The model under review builds one solid part; all positions refer to its coordinate system, in mm. Face numbers are marked on the shaded views. A direction names the side the tool comes from. Coordinates: 2 decimals unless noted, no trailing zeros. Loops run counter-clockwise (first coordinate to the right, second up) from the corner with the lowest first, then second, coordinate; pieces in that order, holes last. Notation, with made-up numbers: M 64,-5 L 73,-5 A35 cw 73,34 Z; hole C 2,8.5 d6. An arc over 180 degrees is marked long. Return JSON: item names as keys, results as strings.
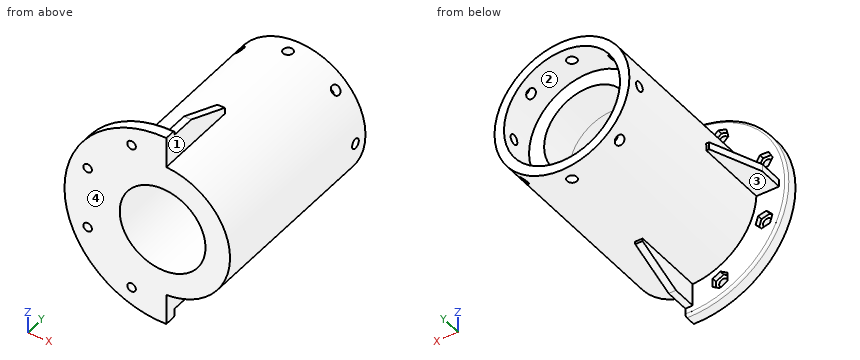
```python
from build123d import *

# Parameters (mm, degrees)
SKETCH1_R                = 27.5
SKETCH1_R_2              = 23.65
BOSS_EXTRUDE1_DEPTH      = 30
SKETCH2_R                = 2
CUT_EXTRUDE1_DEPTH       = 28.5
CIRPATTERN1_COUNT        = 4
CIRPATTERN1_ANGLE        = 135
SKETCH3_R                = 27.5
SKETCH3_R_2              = 23.65
BOSS_EXTRUDE2_DEPTH      = 51
BOSS_EXTRUDE3_DEPTH      = 5
SKETCH6_W                = 3
SKETCH6_H                = 12
SKETCH6_W_2              = 12
SKETCH6_H_2              = 3
BOSS_EXTRUDE4_DEPTH      = 30
CHAMFER1_SIZE            = 20
CHAMFER1_SIZE2           = 8.080524517
CHAMFER1_PART_2_SIZE     = 20
CHAMFER1_PART_2_SIZE2    = 8.080524517
CHAMFER1_PART_3_SIZE     = 20
CHAMFER1_PART_3_SIZE2    = 8.080524517
SKETCH7_R                = 1.75
CUT_EXTRUDE2_DEPTH       = 6.0000001
CUT_EXTRUDE3_DEPTH       = 2
CIRPATTERN2_COUNT        = 4
CIRPATTERN2_ANGLE        = 135
FILLET1_R                = 1
SKETCH9_R                = 26.233260483
SKETCH9_R_2              = 17.5
BOSS_EXTRUDE5_DEPTH      = 15
BOSS_EXTRUDE5_DEPTH_BACK = 51


with BuildPart() as part:
    # Sketch1 → Boss-Extrude1 (new body)
    with BuildSketch(Plane(origin=(0, 0, 0), x_dir=(1, 0, 0), z_dir=(0, 1, 0))):
        Circle(SKETCH1_R)
        Circle(SKETCH1_R_2, mode=Mode.SUBTRACT)
    extrude(amount=BOSS_EXTRUDE1_DEPTH)

    # Sketch2 → Cut-Extrude1 (cut, symmetric)
    with BuildSketch(Plane.XY):
        with Locations((0, 24)):
            Circle(SKETCH2_R)
    cut_extrude1 = extrude(amount=CUT_EXTRUDE1_DEPTH, both=True, mode=Mode.SUBTRACT)

    # CirPattern1: Cut-Extrude1 ×4 about axis
    cirpattern1_axis = Axis((0, 30, 0), (0, 1, 0))
    for i in range(1, CIRPATTERN1_COUNT):
        add(cut_extrude1.rotate(cirpattern1_axis, i * CIRPATTERN1_ANGLE / (CIRPATTERN1_COUNT - 1)), mode=Mode.SUBTRACT)

    # Sketch3 → Boss-Extrude2 (add)
    with BuildSketch(Plane.XZ):
        Circle(SKETCH3_R)
        Circle(SKETCH3_R_2, mode=Mode.SUBTRACT)
    extrude(amount=BOSS_EXTRUDE2_DEPTH)

    # Sketch4 → Boss-Extrude3 (add)
    with BuildSketch(Plane.XZ.offset(51)):
        with BuildLine():
            Line((1.5, 27.459060435), (1.5, 39.971865105))
            ThreePointArc((1.5, 39.971865105), (-40, 0), (1.5, -39.971865105))
            Line((1.5, -39.971865105), (1.5, -27.459060435))
            ThreePointArc((1.5, -27.459060435), (-27.5, 0), (1.5, 27.459060435))
        make_face()
    extrude(amount=-BOSS_EXTRUDE3_DEPTH)

    # Sketch6 → Boss-Extrude4 (add)
    with BuildSketch(Plane(origin=(0, -46, 0), x_dir=(1, 0, 0), z_dir=(0, 1, 0))):
        with Locations((0, 30.644528231)):
            Rectangle(SKETCH6_W, SKETCH6_H)
        with Locations((-30.709825096, -0.28052704)):
            Rectangle(SKETCH6_W_2, SKETCH6_H_2)
        with Locations((0, -32.114539573)):
            Rectangle(SKETCH6_W, SKETCH6_H)
    extrude(amount=BOSS_EXTRUDE4_DEPTH)

    # Chamfer1
    chamfer1_edges = [part.edges().sort_by_distance(p)[0] for p in [
        (0, -16, -36.644528231),
    ]]
    chamfer1_side = [part.faces().sort_by_distance(p)[0] for p in [
        (0, -31, -36.644528231),
    ]]
    chamfer(chamfer1_edges, length=CHAMFER1_SIZE, length2=CHAMFER1_SIZE2, reference=chamfer1_side[0])

    # Chamfer1 part 2
    chamfer1_part_2_edges = [part.edges().sort_by_distance(p)[0] for p in [
        (-36.709825096, -16, 0.28052704),
    ]]
    chamfer1_part_2_side = [part.faces().sort_by_distance(p)[0] for p in [
        (-36.709825096, -31, 0.28052704),
    ]]
    chamfer(chamfer1_part_2_edges, length=CHAMFER1_PART_2_SIZE, length2=CHAMFER1_PART_2_SIZE2, reference=chamfer1_part_2_side[0])

    # Chamfer1 part 3
    chamfer1_part_3_edges = [part.edges().sort_by_distance(p)[0] for p in [
        (0, -16, 38.114539573),
    ]]
    chamfer1_part_3_side = [part.faces().sort_by_distance(p)[0] for p in [
        (0, -31, 38.114539573),
    ]]
    chamfer(chamfer1_part_3_edges, length=CHAMFER1_PART_3_SIZE, length2=CHAMFER1_PART_3_SIZE2, reference=chamfer1_part_3_side[0])

    # Sketch7 → Cut-Extrude2 (cut, through all)
    with BuildSketch(Plane(origin=(0, -46, 0), x_dir=(1, 0, 0), z_dir=(0, 1, 0))):
        with Locations((-12.663510369, 30.572418481)):
            Circle(SKETCH7_R)
    cut_extrude2 = extrude(amount=-CUT_EXTRUDE2_DEPTH, mode=Mode.SUBTRACT)

    # Sketch8 → Cut-Extrude3 (cut)
    with BuildSketch(Plane(origin=(0, -46, 0), x_dir=(1, 0, 0), z_dir=(0, 1, 0))):
        Polygon((-9.561603451, 32.24020348), (-12.556901088, 34.092641172), (-15.658808006, 32.424856172), (-15.765417287, 28.904633481), (-12.770119651, 27.05219579), (-9.668212733, 28.719980789), align=None)
    cut_extrude3 = extrude(amount=-CUT_EXTRUDE3_DEPTH, mode=Mode.SUBTRACT)

    # CirPattern2: Cut-Extrude2, Cut-Extrude3 ×4 about axis
    cirpattern2_axis = Axis((0, 0, 0), (0, 1, 0))
    for i in range(1, CIRPATTERN2_COUNT):
        add(cut_extrude2.rotate(cirpattern2_axis, i * CIRPATTERN2_ANGLE / (CIRPATTERN2_COUNT - 1)), mode=Mode.SUBTRACT)
        add(cut_extrude3.rotate(cirpattern2_axis, i * CIRPATTERN2_ANGLE / (CIRPATTERN2_COUNT - 1)), mode=Mode.SUBTRACT)

    # Fillet1
    fillet1_edges = [part.edges().sort_by_distance(p)[0] for p in [
        (-40, -46, 0),
    ]]
    fillet(fillet1_edges, radius=FILLET1_R)

    # Sketch9 → Boss-Extrude5 (add, two sides)
    with BuildSketch(Plane(origin=(0, 0, 0), x_dir=(1, 0, 0), z_dir=(0, 1, 0))) as boss_extrude5_sk:
        Circle(SKETCH9_R)
        Circle(SKETCH9_R_2, mode=Mode.SUBTRACT)
    extrude(amount=BOSS_EXTRUDE5_DEPTH)
    extrude(boss_extrude5_sk.sketch, amount=-BOSS_EXTRUDE5_DEPTH_BACK)


solid = part.part
```
1. Add section D-D on y = 24. State how many separate pieces and enclosed holes the cut face has, plus the area to 3 significant figures.
Check values:
{"separate pieces": "8", "enclosed holes": "0", "area": "495 mm²"}
2. Add section B-B on y = -39. Give the boundary of the cut face in (x, z).
Check values:
{"outline": "M -36.71,-1.22 L -27.47,-1.22 A27.5 ccw -1.5,-27.46 L -1.5,-36.64 L 1.5,-36.64 L 1.5,-27.46 A27.5 ccw 1.5,27.46 L 1.5,38.11 L -1.5,38.11 L -1.5,27.46 A27.5 ccw -27.44,1.78 L -36.71,1.78 Z; hole C 0,0 d35"}
3. Add section A-A on z = 0. Give the boundary of the cut face in (x, y).
Check values:
{"outline": "M -40,-51 L -17.5,-51 L -17.5,15 L -23.65,15 L -23.65,22 L -27.5,22 L -27.5,-16 L -28.63,-16 L -36.71,-36 L -36.71,-46 L -39,-46 A1 ccw -40,-47 Z; M -27.5,26 L -23.65,26 L -23.65,30 L -27.5,30 Z; M 17.5,-51 L 27.5,-51 L 27.5,22 L 23.65,22 L 23.65,15 L 17.5,15 Z; M 23.65,26 L 27.5,26 L 27.5,30 L 23.65,30 Z"}
4. Add section C-C on x = 8. Give the boundary of the cut face in (y, z), plus the area to 3 significant figures.
Check values:
{"outline": "M -51,-26.31 L 30,-26.31 L 30,-22.26 L 15,-22.26 L 15,-15.56 L -51,-15.56 Z; M -51,15.56 L 15,15.56 L 15,22.26 L 30,22.26 L 30,26.31 L -51,26.31 Z", "area": "1,540 mm²"}
5. Insertion check: pin 1 Ø3 at (y, z) = (14, 17) entering from +X; pin 2 Ø3 at (x, y) = (-32, -30) entering from +Z; pin 3 Ø4.5 at (x, z) = (-12.66, 30.57) entering from +Y. Each pin has a flat end and moves straight along its axis. Give the tip position at first contact, or say it passes through.
Check values:
{"pin 1": "x = 22.72", "pin 2": "z = 1.78", "pin 3": "y = -48"}
6. Machinability: for the marked faces 1, 2, 3 and 4, which of the approach directions +Z, -Z, +X, -X, +Y, -Y give a long, thin tool a straight path to every point of the face, cutting with its end or side? Answer none if there is none.
Check values:
{"face 1": "+Z, +X, +Y, -Y", "face 2": "+Y", "face 3": "-Z, -X, +Y", "face 4": "+Z, -Z, +X, -X, -Y"}
7. To check wall thickness, follow line 1 (Z direction, x = 0, y = 10.75); line 2 (Z direction, x = 11.5, y = 18); line 3 (X direction, y = -19.5, z = 9.5). State the ranges of each line that lie inside material, in increasing order.
Check values:
{"line 1": "-27.5 to -17.5, 17.5 to 27.5", "line 2": "-24.98 to -20.67, 20.67 to 24.98", "line 3": "-25.81 to -14.7, 14.7 to 25.81"}
